Input: part model. Units: mm. Frame: model coordinates. Face numbers are marked on the shaded views. A direction names the side the tool comes from. Coordinates: 2 decimals unless noted, no trailing zeros. Loops run counter-clockwise (first coordinate to the right, second up) from the corner with the lowest first, then second, coordinate; pieces in that order, holes last. Notation, with made-up numbers: (-2, 3) -> (18, 3) arc R32 cw to (18, 37) -> close; hole circle Ø1 at (-24, 57.25). An arc over 180 degrees is marked (long way). Answer as a JSON object with one key per item and string values.
from build123d import *

# Parameters (mm, degrees)
SKETCH1_W           = 83.82
SKETCH1_H           = 12.7
SKETCH1_R           = 2.286
BOSS_EXTRUDE1_DEPTH = 25.4
SKETCH2_R           = 2.286
CUT_EXTRUDE1_DEPTH  = 12.7
FILLET1_R           = 2.54
SKETCH3_W           = 71.12
SKETCH3_H           = 19.05
CUT_EXTRUDE2_DEPTH  = 89.499957062


with BuildPart() as part:
    # Sketch1 → Boss-Extrude1 (new body)
    with BuildSketch(Plane(origin=(0, 0, 0), x_dir=(1, 0, 0), z_dir=(0, 1, 0))):
        with Locations((41.91, 6.35)):
            Rectangle(SKETCH1_W, SKETCH1_H)
        with Locations(Location((6.35, 6.35, 0), (0, 0, 90))):
            Circle(SKETCH1_R, mode=Mode.SUBTRACT)
        with Locations(Location((47.659178157, 6.35, 0), (0, 0, 90))):
            Circle(SKETCH1_R, mode=Mode.SUBTRACT)
    extrude(amount=BOSS_EXTRUDE1_DEPTH)

    # Sketch2 → Cut-Extrude1 (cut)
    with BuildSketch(Plane.XY):
        with Locations((77.47, 19.05)):
            Circle(SKETCH2_R)
    extrude(amount=-CUT_EXTRUDE1_DEPTH, mode=Mode.SUBTRACT)

    # Fillet1
    fillet1_edges = [part.edges().sort_by_distance(p)[0] for p in [
        (0, 12.7, -12.7),
        (83.82, 12.7, -12.7),
        (83.82, 12.7, 0),
        (0, 12.7, 0),
    ]]
    fillet(fillet1_edges, radius=FILLET1_R)

    # Sketch3 → Cut-Extrude2 (cut, through all)
    with BuildSketch(Plane.XY):
        with Locations((35.56, 15.875)):
            Rectangle(SKETCH3_W, SKETCH3_H)
    extrude(amount=-CUT_EXTRUDE2_DEPTH, mode=Mode.SUBTRACT)


solid = part.part
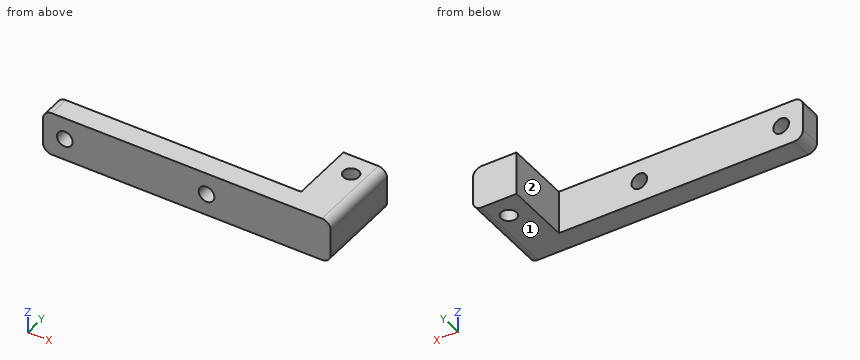
1. Pin query (flat end, axial travel): P1, Ø6, axis at x = 6.35, z = -6.35, coming from the +Y side; P2, Ø6.5, axis at y = 17, z = -5, coming from the -X side. Return the tip coordinate at first contact, or that it passes through.
Reply:
{"P1": "stops at y = 6.35", "P2": "stops at x = 71.12"}
2. Section query B-B (z = -6.35). Return loops of the section in (x, y), plus the area to 3 significant figures.
Reply:
{"outline": "(0, 0) -> (4.06, 0) -> (4.06, 6.35) -> (0, 6.35) -> close; (8.64, 0) -> (45.37, 0) -> (45.37, 6.35) -> (8.64, 6.35) -> close; (49.95, 0) -> (83.82, 0) -> (83.82, 25.4) -> (71.12, 25.4) -> (71.12, 6.35) -> (49.95, 6.35) -> close; hole circle Ø4.57 at (77.47, 19.05)", "area": "700 mm2"}
3. Line query: line 1 along X through (y, z) = (4, -6.35); line 2 along Y through (x, z) = (77.47, -9.75); line 3 along Y through (x, z) = (17.5, -2.5). Output: solid intervals per line, ascending.
Reply:
{"line 1": "x = 0 to 4.06, 8.64 to 45.37, 49.95 to 83.82", "line 2": "y = 0 to 16.76, 21.34 to 25.4", "line 3": "y = 0 to 6.35"}
4. Access query for the marked faces 1 and 2. Directions: +Z, -Z, +X, -X, +Y, -Y. A direction counts if a zero-diameter tool reaches every point of the face in a straight line with its end or side. Return the directions, or none.
Reply:
{"face 1": "-Z, +X, -X, +Y, -Y", "face 2": "+Z, -Z, -X, +Y"}
5. Section query A-A (x = 77.47). Return loops of the section in (y, z), plus the area to 3 significant figures.
Reply:
{"outline": "(0, -12.7) -> (16.76, -12.7) -> (16.76, 0) -> (0, 0) -> close; (21.34, -12.7) -> (25.4, -12.7) -> (25.4, 0) -> (21.34, 0) -> close", "area": "265 mm2"}
6. Section query C-C (y = 19.05). Return loops of the section in (x, z), plus the area to 3 significant figures.
Reply:
{"outline": "(71.12, -12.7) -> (75.18, -12.7) -> (75.18, 0) -> (71.12, 0) -> close; (79.76, -12.7) -> (81.28, -12.7) arc R2.54 ccw to (83.82, -10.16) -> (83.82, -2.54) arc R2.54 ccw to (81.28, 0) -> (79.76, 0) -> close", "area": "100 mm2"}
7. Section query D-D (z = -11). Return loops of the section in (x, y).
Reply:
{"outline": "(0.14, 0) -> (83.68, 0) -> (83.68, 25.4) -> (71.12, 25.4) -> (71.12, 6.35) -> (0.14, 6.35) -> close; hole circle Ø4.57 at (77.47, 19.05)"}
